The figure shows three views and two pictorial views of one solid part (mm, origin at its lowest corner). Answer the questions. A direction names the side the tool comes from. Round coordinates to 2 decimals unless told otherwise and drop trailing zeros. Order: outer loops, then holes, each group sorted by start corner. A loop starts at its lowest first (then second) coordinate and runs counter-clockwise, first axis right, second up. Notation, with made-up numbers: M 73,-7.5 L 111,-7.5 A28 ccw 111,21.5 Z; hole C -17,5.25 d2. An arc over 180 degrees is marked long. Return JSON: item names as keys, results as strings.
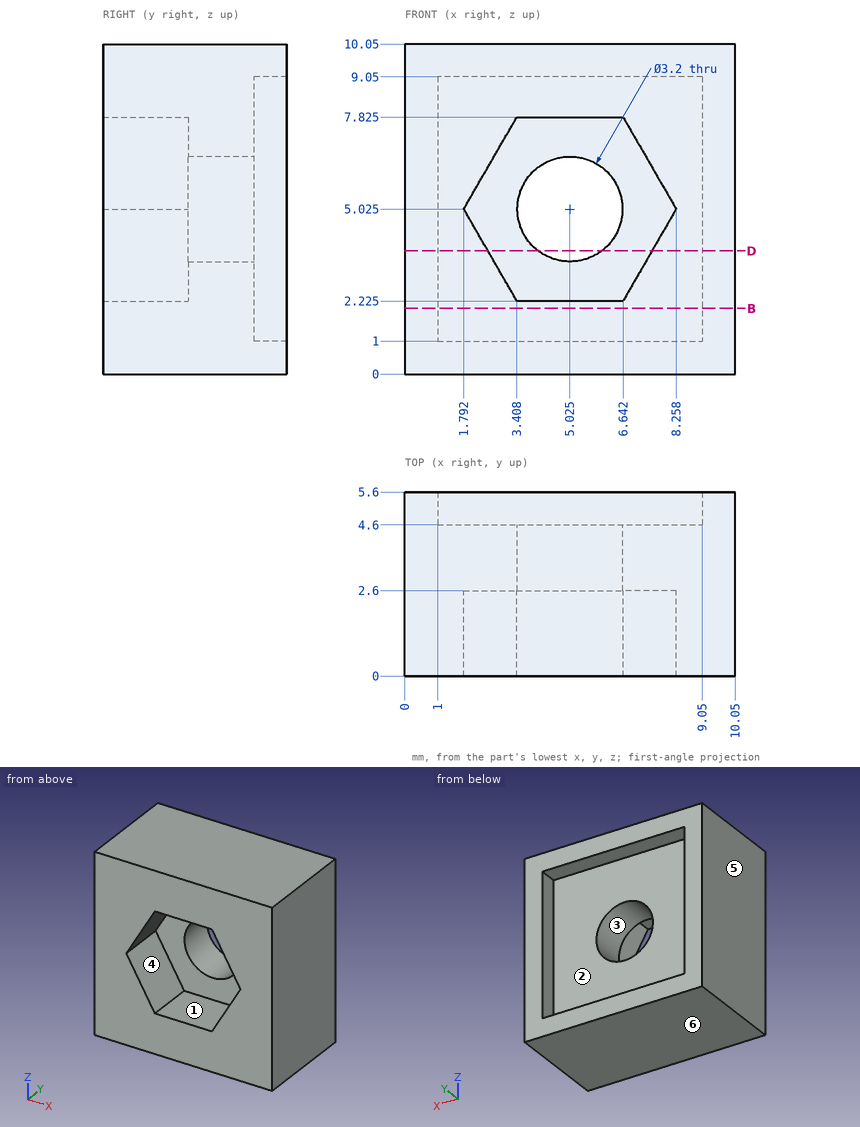
Item 1: Which of the six approach directions +Z, -Z, +X, -X, +Y, -Y give full straight-line access (tool end or side, diameter ignored) to the marked faces 1, 2 and 3?
Output:
{"face 1": "-Y", "face 2": "+Y", "face 3": "+Y, -Y"}
Item 2: Each of these flat-tipped pins is pushed along its axis until it touches: pin 1 (1.7 mm diameter, centred on x = 5.5, z = 4, fed in from -Y); pin 2 (4 mm diameter, centred on x = 5.5, z = 3.5, fed in from +Y). Where does it stop, or does it pass through?
Output:
{"pin 1": "stops at y = 2.6", "pin 2": "stops at y = 4.6"}
Item 3: Find section B-B (z = 2). Determine the outline of the cut face in (x, y).
Output:
{"outline": "M 0,0 L 10.05,0 L 10.05,5.6 L 9.05,5.6 L 9.05,4.6 L 1,4.6 L 1,5.6 L 0,5.6 Z"}
Item 4: Find section D-D (z = 3.75). Determine the outline of the cut face in (x, y).
Output:
{"outline": "M 0,0 L 2.53,0 L 2.53,2.6 L 4.06,2.6 L 4.06,4.6 L 1,4.6 L 1,5.6 L 0,5.6 Z; M 5.99,2.6 L 7.52,2.6 L 7.52,0 L 10.05,0 L 10.05,5.6 L 9.05,5.6 L 9.05,4.6 L 5.99,4.6 Z"}
Item 5: The mould has two halves that part along Z. Classify the marked faces 4, 5 and 6: pulls with the +Z half, pulls with the -Z half, needs draft (parallel to the pull), parting line crosses it, or undercut.
Output:
{"face 4": "undercut", "face 5": "needs draft", "face 6": "pulls with the -Z half"}
Item 6: Consider line 1 along Z through (x, y) = (7.75, 5.2); line 2 along Y through (x, z) = (5, 2.75); line 3 along Y through (x, z) = (9, 3.25). Determine where each line is inside the solid, lowest interval first. Write a range as [from, to].
Output:
{"line 1": "z = [0, 1], [9.05, 10.05]", "line 2": "y = [2.6, 4.6]", "line 3": "y = [0, 4.6]"}
